Here's how the part is built. I have some questions about the finished solid (model axes, mm). Face numbers are marked on the shaded views. A direction names the side the tool comes from. Coordinates: 2 decimals unless noted, no trailing zeros. Write each loop counter-clockwise with the first axis right and the second up, starting at its lowest first coordinate (ties: lowest second). Pieces come first, ordered by that corner, then holes. Notation, with made-up numbers: (53.25, 71.25) -> (65.25, 71.25) arc R16 ccw to (65.25, 95.25) -> close; hole circle Ø7 at (23, -7.75). An arc over 180 degrees is marked (long way). Put each result on its own line as item: value. Start each with the question number.
Item 1: I want a section at D-D, the plane y = 11.5. List the corners of the cut face in (x, z) for me, then the cut area to 4 significant figures.
Item 2: If we mould it in two halves opening along Z, with no side actions, what happens to the marked faces 3, 4, 5 and 6? For each: released by +Z, released by -Z, zero draft, split by the parting line, or undercut.
Item 3: I want a section at C-C, the plane x = 29. List the corners of the cut face in (y, z) for me, then the cut area to 3 significant figures.
Item 4: For pin 1 (6 mm diameter, centred on x = 0, z = 10, fed in from +Y); pin 2 (16 mm diameter, centred on x = 0, z = -10, fed in from +Y); pin 3 (3 mm diameter, centred on y = 12.5, z = 4.5, fed in from +X), each with a flat end and sliding along its axis, tell me the tip position at first contact or that it passes through.
Item 5: On a 3-axis mill with a long thin cutter (end or side, diameter ignored), from which of +Z, -Z, +X, -X, +Y, -Y can I reach the whole of each face in a straight line? I mean the marked faces 1 and 2. Say none if no direction works.
Item 6: I want a section at A-A, the plane z = 10. List the corners of the cut face in (x, y) for me.
Item 7: I want a section at B-B, the plane z = -4. List the corners of the cut face in (x, y) for me.
Item 8: I need wall thicknesses on line 1 (Z direction, x = 0, y = 2.35); line 2 (Z direction, x = 0, y = 3.95); line 3 (Z direction, x = 14, y = 7.5). Which ranges of each line are inside material? Lowest first, please. Write a range as [from, to].
from build123d import *

# Parameters (mm, degrees)
SKETCH3_W               = 73.5
SKETCH3_H               = 54
BOSS_EXTRUDE2_DEPTH     = 5
BOSS_EXTRUDE4_DEPTH     = 15
SKETCH6_R               = 5
SKETCH6_R_2             = 2.5
CUT_EXTRUDE4_DEPTH      = 2
SKETCH1_R               = 2.5
CUT_EXTRUDE5_DEPTH      = 10
CUT_EXTRUDE5_DEPTH_BACK = 1
SKETCH1_7_R             = 2.5
CUT_EXTRUDE6_DEPTH      = 10


with BuildPart() as part:
    # Sketch3 → Boss-Extrude2 (new body)
    with BuildSketch(Plane(origin=(0, 0, 0), x_dir=(1, 0, 0), z_dir=(0, 1, 0))):
        Rectangle(SKETCH3_W, SKETCH3_H)
    extrude(amount=BOSS_EXTRUDE2_DEPTH)

    # Sketch4 → Boss-Extrude4 (add)
    with BuildSketch(Plane(origin=(0, 0, 0), x_dir=(1, 0, 0), z_dir=(0, 1, 0))):
        Polygon((36.75, 32), (-41.75, 32), (-41.75, -32), (36.75, -32), (36.75, -27), (-36.75, -27), (-36.75, 27), (36.75, 27), align=None)
    extrude(amount=BOSS_EXTRUDE4_DEPTH)

    # Sketch6 → Cut-Extrude4 (cut)
    with BuildSketch(Plane(origin=(0, 5, 0), x_dir=(1, 0, 0), z_dir=(0, 1, 0))):
        with Locations((0, 10)):
            Circle(SKETCH6_R)
        with Locations((0, 10)):
            Circle(SKETCH6_R_2, mode=Mode.SUBTRACT)
        with Locations((0, -10)):
            Circle(SKETCH6_R)
        with Locations((0, -10)):
            Circle(SKETCH6_R_2, mode=Mode.SUBTRACT)
    extrude(amount=-CUT_EXTRUDE4_DEPTH, mode=Mode.SUBTRACT)

    # Sketch1 → Cut-Extrude5 (cut, two sides)
    with BuildSketch(Plane(origin=(0, 0, 0), x_dir=(1, 0, 0), z_dir=(0, 1, 0))) as cut_extrude5_sk:
        with Locations((0, 10)):
            Circle(SKETCH1_R)
    extrude(amount=CUT_EXTRUDE5_DEPTH, mode=Mode.SUBTRACT)
    extrude(cut_extrude5_sk.sketch, amount=-CUT_EXTRUDE5_DEPTH_BACK, mode=Mode.SUBTRACT)

    # Sketch1<7> → Cut-Extrude6 (cut)
    with BuildSketch(Plane(origin=(0, 0, 0), x_dir=(1, 0, 0), z_dir=(0, 1, 0))):
        with Locations((0, -10)):
            Circle(SKETCH1_7_R)
    extrude(amount=CUT_EXTRUDE6_DEPTH, mode=Mode.SUBTRACT)


solid = part.part
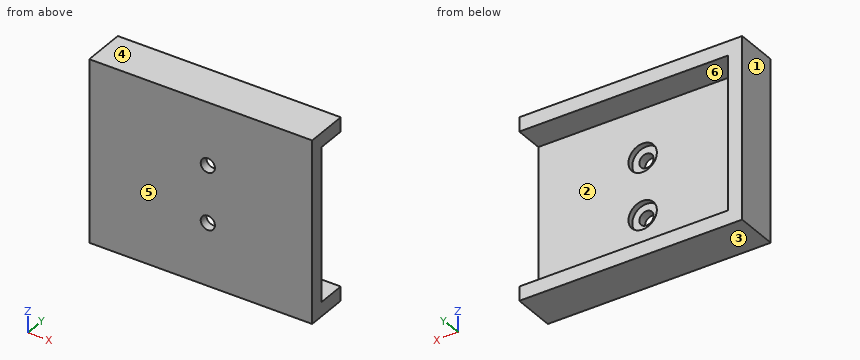
Calculated:
1. outline: (-41.75, -32) -> (36.75, -32) -> (36.75, -27) -> (-36.75, -27) -> (-36.75, 27) -> (36.75, 27) -> (36.75, 32) -> (-41.75, 32) -> close
1. area: 1,055 mm2
2. face 3: released by -Z
2. face 4: released by +Z
2. face 5: zero draft
2. face 6: undercut
3. outline: (0, -32) -> (15, -32) -> (15, -27) -> (5, -27) -> (5, 27) -> (15, 27) -> (15, 32) -> (0, 32) -> close
3. area: 420 mm2
4. pin 1: stops at y = 3
4. pin 2: stops at y = 5
4. pin 3: stops at x = -36.75
5. face 1: +Z, -Z, -X, +Y, -Y
5. face 2: +X, +Y
6. outline: (-41.75, 0) -> (-2.5, 0) -> (-2.5, 3) -> (-5, 3) -> (-5, 5) -> (-36.75, 5) -> (-36.75, 15) -> (-41.75, 15) -> close; (2.5, 0) -> (36.75, 0) -> (36.75, 5) -> (5, 5) -> (5, 3) -> (2.5, 3) -> close
7. outline: (-41.75, 0) -> (36.75, 0) -> (36.75, 5) -> (-36.75, 5) -> (-36.75, 15) -> (-41.75, 15) -> close
8. line 1: z = [-32, -12.5], [-7.5, 7.5], [12.5, 32]
8. line 2: z = [-32, -15], [-5, 5], [15, 32]
8. line 3: z = [-32, -27], [27, 32]
